```python
from build123d import *

# Parameters (mm, degrees)
SKETCH1_R           = 10
SKETCH1_R_2         = 5
SKETCH4_R           = 15
SKETCH4_R_2         = 5
BOSS_EXTRUDE1_DEPTH = 3
SKETCH5_W           = 3
SKETCH5_H           = 3
CUT_EXTRUDE1_DEPTH  = 3


with BuildPart() as part:
    # Sweep1: sweep along a path in Sketch3
    with BuildLine(Plane(origin=(0, 0, 0), x_dir=(0, 0, -1), z_dir=(1, 0, 0))) as sweep1_path:
        ThreePointArc((0, 0), (-7.533795299, 3.120600189), (-10.654395489, 10.654395489))
    # Sketch1 → Sweep1 (sweep)
    with BuildSketch(Plane.XY):
        Circle(SKETCH1_R)
        Circle(SKETCH1_R_2, mode=Mode.SUBTRACT)
    sweep(path=sweep1_path.line)

    # Sketch4 → Boss-Extrude1 (add)
    with BuildSketch(Plane(origin=(0, 0, 0), x_dir=(-1, 0, 0), z_dir=(0, 0, -1))):
        Circle(SKETCH4_R)
        Circle(SKETCH4_R_2, mode=Mode.SUBTRACT)
    extrude(amount=BOSS_EXTRUDE1_DEPTH)

    # Sketch5 → Cut-Extrude1 (cut)
    with BuildSketch(Plane(origin=(0, 10.654395489, 0), x_dir=(1, 0, 0), z_dir=(0, 1, 0))):
        with Locations((0, -3.154395489)):
            Rectangle(SKETCH5_W, SKETCH5_H)
        with Locations((0, -18.154395489)):
            Rectangle(SKETCH5_W, SKETCH5_H)
    extrude(amount=-CUT_EXTRUDE1_DEPTH, mode=Mode.SUBTRACT)


solid = part.part
```
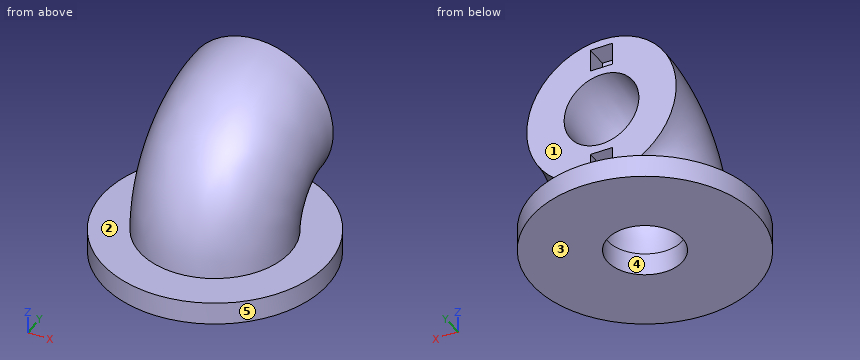
Can you work these out from the model? Positions are in its coordinate system, mm. Face numbers are marked on the shaded views. A direction names the side the tool comes from. Give positions to 0.01 mm unless a question says otherwise; leave off trailing zeros. Write each loop counter-clockwise with the first axis right and the second up, starting at its lowest first coordinate (ties: lowest second). Pieces come first, ordered by that corner, then holes. Notation, with made-up numbers: (-1, 85) - (23, 85) arc R20 ccw to (23, 97) - close; hole circle Ø6 at (56.25, 35). An arc over 180 degrees is marked (long way). Write item = value, one per line. Start each with the question number.
1. Imagine slicing it at B-B (x = 7). Please give me the cut outline in (y, z).
2. Imagine slicing it at C-C (x = 12). Please give me the cut outline in (y, z), and give its area (3 significant figures).
3. Please list where these lines run through material, in increasing order: line 1 (Y direction, x = 0, z = -2.1); line 2 (Z direction, x = 4.5, y = 7.5); line 3 (Z direction, x = -0.75, y = 6.25).
4. Imagine slicing it at A-A (x = 0). Please give me the cut outline in (y, z), and give its area (3 significant figures).
5. Thinking about a two-plate mould opening in Z: for the marked faces 1, 2 and 3, which applies, released by +Z, released by -Z, zero draft, split by the parting line, or undercut?
6. For pin 1 (3 mm diameter, centred on x = 0.5, y = 1, fed in from +Z); pin 2 (1.5 mm diameter, centred on x = 0.5, y = 9.5, fed in from +Z); pin 3 (0.9 mm diameter, centred on y = 10, z = 3.5, fed in from +X), each with a flat end and sliding along its axis, tell me the tip position at first contact or that it passes through.
7. On a 3-axis mill with a long thin cutter (end or side, diameter ignored), from which of +Z, -Z, +X, -X, +Y, -Y can I reach the whole of each face in a straight line? I mean the marked faces 4 and 5. Say none if no direction works.
Worked answers:
q1.outline = (-13.27, -3) - (13.27, -3) - (13.27, 0) - (7.14, 0) arc R3.51 cw to (10.65, 3.51) - (10.65, 17.8) arc R17.8 ccw to (-7.14, 0) - (-13.27, 0) - close
q2.outline = (-9, -3) - (9, -3) - (9, 0) - (-9, 0) - close
q2.area = 54.0 mm2
q3.line_1 = -15 to -5, 5 to 15
q3.line_2 = -3 to 7.87, 12.44 to 19.33
q3.line_3 = -3 to 3.64, 14.96 to 20.15
q4.outline = (-15, -3) - (-5, -3) - (-5, 0) arc R15.65 cw to (10.65, 15.65) - (10.65, 16.65) - (7.65, 16.65) - (7.65, 19.65) - (10.65, 19.65) - (10.65, 20.65) arc R20.65 ccw to (-10, 0) - (-15, 0) - close; (5, -3) - (15, -3) - (15, 0) - (10, 0) arc R0.65 cw to (10.65, 0.65) - (10.65, 1.65) - (7.65, 1.65) - (7.65, 4.65) - (10.65, 4.65) - (10.65, 5.65) arc R5.65 ccw to (5, 0) - close
q4.area = 209 mm2
q5.face_1 = zero draft
q5.face_2 = undercut
q5.face_3 = released by -Z
q6.pin_1 = 18.97
q6.pin_2 = 20.65
q6.pin_3 = 7.47
q7.face_4 = -Z
q7.face_5 = +Z, -Z
